```python
from build123d import *

# Parameters (mm, degrees)
SKETCH1_W           = 200
SKETCH1_H           = 200
BOSS_EXTRUDE2_DEPTH = 200
SKETCH3_R           = 100
BOSS_EXTRUDE3_DEPTH = 100
BOSS_EXTRUDE4_DEPTH = 50


with BuildPart() as part:
    # Sketch1 → Boss-Extrude2 (new body)
    with BuildSketch(Plane(origin=(0, 0, 0), x_dir=(1, 0, 0), z_dir=(0, 1, 0))):
        Rectangle(SKETCH1_W, SKETCH1_H)
    extrude(amount=BOSS_EXTRUDE2_DEPTH)

    # Sketch3 → Boss-Extrude3 (add)
    with BuildSketch(Plane(origin=(0, 200, 0), x_dir=(1, 0, 0), z_dir=(0, 1, 0))):
        with Locations(Location((0, 0, 0), (0, 0, 270))):
            Circle(SKETCH3_R)
    extrude(amount=BOSS_EXTRUDE3_DEPTH)

    # Sketch4 → Boss-Extrude4 (add)
    with BuildSketch(Plane(origin=(0, 300, 0), x_dir=(1, 0, 0), z_dir=(0, 1, 0))):
        Polygon((0, 100), (-86.602540378, -50), (86.602540378, -50), align=None)
    extrude(amount=BOSS_EXTRUDE4_DEPTH)


solid = part.part
```
Here's how the part is built. I have some questions about the finished solid (model axes, mm). A direction names the side the tool comes from. Coordinates: 2 decimals unless noted, no trailing zeros. Write each loop counter-clockwise with the first axis right and the second up, starting at its lowest first coordinate (ties: lowest second). Pieces come first, ordered by that corner, then holes. Notation, with made-up numbers: (42.25, 51.5) -> (65.25, 51.5) arc R25 cw to (65.25, 66.5) -> close; hole circle Ø6 at (26.5, 51.5). An arc over 180 degrees is marked (long way). Use a Markdown table: item, result. Add a question column.
(1) I'm going to push flat-ended pins straight in: P1, Ø15, axis at x = 2, z = 84, coming from the +Y side; P2, Ø15, axis at x = 36.5, y = 336.5, coming from the +Z side; P3, Ø3, axis at y = 252.5, z = -30.5, coming from the -X side. Where does each tip first touch, or does it pass through?
(2) If we section it at A-A, the plane x = 30: Write out the boundary of the cut face in (y, z).
(3) If we section it at C-C, the plane y = 212.5: Write out the boundary of the cut face in (x, z).
(4) Please list where these lines run through material, in increasing order: line 1 (Y direction, x = 85, z = 46.5); line 2 (Y direction, x = 91, z = 70); line 3 (Z direction, x = -44, y = 311.5).
(5) If we section it at B-B, the plane z = -83.5: Write out the boundary of the cut face in (x, y) (3 decimals).
(6) For faces 1 (the flat face through (-42.695, 324.65, -26.05)), 2 (the flat face through (43.907, 324.65, -23.95)), 3 (the cylindrical face through (30.04, 249.3, 95.38)), which set-ups out of +Z, -Z, +X, -X, +Y, -Y let a thin tool reach every point of the face, with its end or its side?
Outcome:
| question | item | result |
|---|---|---|
| 1 | P1 | stops at y = 300 |
| 1 | P2 | stops at z = 50 |
| 1 | P3 | stops at x = -95.7 |
| 2 | outline | (0, -100) -> (200, -100) -> (200, -95.39) -> (300, -95.39) -> (300, -48.04) -> (350, -48.04) -> (350, 50) -> (300, 50) -> (300, 95.39) -> (200, 95.39) -> (200, 100) -> (0, 100) -> close |
| 3 | outline | circle Ø200 at (0, 0) |
| 4 | line 1 | y = 0 to 300 |
| 4 | line 2 | y = 0 to 200 |
| 4 | line 3 | z = -23.79 to 50 |
| 5 | outline | (-100, 0) -> (100, 0) -> (100, 200) -> (55.025, 200) -> (55.025, 300) -> (9.526, 300) -> (9.526, 350) -> (-9.526, 350) -> (-9.526, 300) -> (-55.025, 300) -> (-55.025, 200) -> (-100, 200) -> close |
| 6 | face 1 | -Z, -X, +Y |
| 6 | face 2 | -Z, +X, +Y |
| 6 | face 3 | +Y |
